Source: CAD feature listing. Evaluate the final solid. Frame: model axes, mm. A direction names the side the tool comes from. Coordinates: 2 decimals unless noted, no trailing zeros. Loops run counter-clockwise (first coordinate to the right, second up) from the corner with the lowest first, then second, coordinate; pieces in that order, holes last.
Item 1: Pin query (flat end, axial travel): pin 1 Ø1.5 at (y, z) = (7.5, -13) entering from -X; pin 2 Ø10 at (x, y) = (60, 7.5) entering from -Z; pin 3 Ø3.5 at (x, z) = (7, 6.5) entering from +Y. Return the tip coordinate at first contact, or that it passes through.
Item 2: Section query C-C, the plane z = 7.3. Return the cut outline in (x, y), then the cut area to 3 significant figures.
Item 3: Section query A-A, the plane y = 0. Return the cut outline in (x, z), then the cut area to 3 significant figures.
Item 4: Section query D-D, the plane x = 58.5. Return the cut outline in (y, z), then the cut area to 3 significant figures.
Item 5: Reachability of faces 1 (the cylindrical face through (18.819, -0.264, 13.294)), 2 (the flat face through (45.2, 7, 15)), 3 (the cylindrical face through (34.3, 15.43, -9.84)) from +Z, -Z, +X, -X, +Y, -Y: full face, straight path, thin tool, end or side. Return the list, or none.
Item 6: Pull-direction query (Y, two-part tool) for faces 4 (the flat face through (28.7, 8, 13)), 5 (the flat face through (68.2, -7, 8)), 6 (the flat face through (6, 2.5, 7)), 7 (the cylindrical face through (56.54, 16.26, 2.13)); classes: +Y half, -Y half, draft (parallel to the pull), parting line (faces both ways), or undercut.
Item 7: Line query: probe 1 along Y at (x, z) = (25, 0); probe 2 along Z at (x, y) = (26, -7); probe 3 along X at (y, z) = (-6, 13). Output: solid intervals per line, ascending.
Item 8: Section query B-B, the plane x = 27. Return the cut outline in (y, z).
```python
from build123d import *

# Parameters (mm, degrees)
SKETCH_1_R               = 3
EXTRUDE_1_DEPTH          = 13.8
SKETCH_2_R               = 6
EXTRUDE_2_DEPTH          = 9.9
SKETCH_3_R               = 18.3
EXTRUDE_3_DEPTH          = 21.5
SKETCH_4_R               = 16.4
EXTRUDE_4_DEPTH          = 23
SKETCH_5_R               = 10
EXTRUDE_5_DEPTH          = 5
CUT_EXTRUDE_1_DEPTH      = 11.5
SKETCH_7_R               = 1.5
CUT_EXTRUDE_2_DEPTH      = 5
PATTERN_CIRCULAR_1_COUNT = 6
SKETCH_8_R               = 8.963335845
CUT_EXTRUDE_3_DEPTH      = 23.7
SKETCH_9_R               = 6
EXTRUDE_6_DEPTH          = 9.9
SKETCH_10_R              = 3
EXTRUDE_7_DEPTH          = 13.8
CUT_EXTRUDE_4_DEPTH      = 11.5


with BuildPart() as part:
    # 草图1 → 凸台-拉伸1 (new body)
    with BuildSketch(Plane(origin=(0, 0, 0), x_dir=(0, 0, -1), z_dir=(1, 0, 0))):
        with Locations(Location((0, 0, 0), (0, 0, 180))):
            Circle(SKETCH_1_R)
    extrude(amount=EXTRUDE_1_DEPTH)

    # 草图2 → 凸台-拉伸2 (add)
    with BuildSketch(Plane(origin=(13.8, 0, 0), x_dir=(0, 0, -1), z_dir=(1, 0, 0))):
        Circle(SKETCH_2_R)
    extrude(amount=EXTRUDE_2_DEPTH)

    # 草图3 → 凸台-拉伸3 (add)
    with BuildSketch(Plane(origin=(23.7, 0, 0), x_dir=(0, 0, -1), z_dir=(1, 0, 0))):
        Circle(SKETCH_3_R)
    extrude(amount=EXTRUDE_3_DEPTH)

    # 草图4 → 凸台-拉伸4 (add)
    with BuildSketch(Plane(origin=(45.2, 0, 0), x_dir=(0, 0, -1), z_dir=(1, 0, 0))):
        Circle(SKETCH_4_R)
    extrude(amount=EXTRUDE_4_DEPTH)

    # 草图5 → 凸台-拉伸5 (add)
    with BuildSketch(Plane(origin=(68.2, 0, 0), x_dir=(0, 0, -1), z_dir=(1, 0, 0))):
        Circle(SKETCH_5_R)
    extrude(amount=EXTRUDE_5_DEPTH)

    # 草图6 → 切除-拉伸1 (cut)
    with BuildSketch(Plane.ZY):
        Polygon((-1.658312395, 2.5), (1.658312395, 2.5), (1.914814447, 4.033173691), (-2.453659142, 4.033173691), align=None)
    extrude(amount=-CUT_EXTRUDE_1_DEPTH, mode=Mode.SUBTRACT)

    # 草图7 → 切除-拉伸2 (cut)
    with BuildSketch(Plane.ZY.offset(-23.7)):
        with Locations((0, 15.5)):
            Circle(SKETCH_7_R)
    cut_extrude_2 = extrude(amount=-CUT_EXTRUDE_2_DEPTH, mode=Mode.SUBTRACT)

    # 阵列(圆周)1: 切除-拉伸2 ×6 about axis
    pattern_circular_1_axis = Axis((0, 0, 0), (1, 0, 0))
    for i in range(1, PATTERN_CIRCULAR_1_COUNT):
        add(cut_extrude_2.rotate(pattern_circular_1_axis, i * 360 / PATTERN_CIRCULAR_1_COUNT), mode=Mode.SUBTRACT)

    # 草图8 → 切除-拉伸3 (cut)
    with BuildSketch(Plane.ZY):
        Circle(SKETCH_8_R)
    extrude(amount=-CUT_EXTRUDE_3_DEPTH, mode=Mode.SUBTRACT)

    # 草图9 → 凸台-拉伸6 (add)
    with BuildSketch(Plane.ZY.offset(-23.7)):
        with Locations(Location((7.3, 0, 0), (0, 0, 180))):
            Circle(SKETCH_9_R)
    extrude(amount=EXTRUDE_6_DEPTH)

    # 草图10 → 凸台-拉伸7 (add)
    with BuildSketch(Plane.ZY.offset(-13.8)):
        with Locations(Location((7.3, 0, 0), (0, 0, 180))):
            Circle(SKETCH_10_R)
    extrude(amount=EXTRUDE_7_DEPTH)

    # 草图11 → 切除-拉伸4 (cut)
    with BuildSketch(Plane.ZY):
        Polygon((5.641687605, 2.5), (8.958312395, 2.5), (9.936132203, 4.4850308), (5.641687605, 3.798836175), align=None)
    extrude(amount=-CUT_EXTRUDE_4_DEPTH, mode=Mode.SUBTRACT)


solid = part.part
```
Verdict:
1. pin 1: stops at x = 28.7
1. pin 2: stops at z = -16.21
1. pin 3: stops at y = 2.5
2. outline: (0, -3) - (13.8, -3) - (13.8, -6) - (23.7, -6) - (23.7, -16.78) - (45.2, -16.78) - (45.2, -14.69) - (68.2, -14.69) - (68.2, -6.83) - (73.2, -6.83) - (73.2, 6.83) - (68.2, 6.83) - (68.2, 14.69) - (45.2, 14.69) - (45.2, 16.78) - (23.7, 16.78) - (23.7, 6) - (13.8, 6) - (13.8, 3) - (11.5, 3) - (11.5, 2.5) - (0, 2.5) - close
2. area: 1,660 mm2
3. outline: (0, 4.3) - (13.8, 4.3) - (13.8, 1.3) - (23.7, 1.3) - (23.7, -18.3) - (45.2, -18.3) - (45.2, -16.4) - (68.2, -16.4) - (68.2, -10) - (73.2, -10) - (73.2, 10) - (68.2, 10) - (68.2, 16.4) - (45.2, 16.4) - (45.2, 18.3) - (23.7, 18.3) - (23.7, 13.3) - (13.8, 13.3) - (13.8, 10.3) - (0, 10.3) - close
3. area: 1,840 mm2
4. outline: circle Ø32.8 at (0, 0)
4. area: 845 mm2
5. face 1: -X
5. face 2: +X
5. face 3: +X, -X
6. face 4: undercut
6. face 5: draft
6. face 6: +Y half
6. face 7: parting line
7. probe 1: y = -18.3 to -17, -14 to 14, 17 to 18.3
7. probe 2: z = -16.91 to -14.72, -12.12 to 12.12, 14.72 to 16.91
7. probe 3: x = 23.7 to 68.2
8. outline: circle Ø36.6 at (0, 0); hole circle Ø3 at (-15.5, 0); hole circle Ø3 at (-7.75, -13.42); hole circle Ø3 at (-7.75, 13.42); hole circle Ø3 at (7.75, -13.42); hole circle Ø3 at (7.75, 13.42); hole circle Ø3 at (15.5, 0)
